Input: part model. Units: mm. Frame: model coordinates. A direction names the side the tool comes from. Coordinates: 2 decimals unless noted, no trailing zeros. Write each loop counter-clockwise with the first axis right and the second up, starting at its lowest first coordinate (ties: lowest second). Pieces come first, ordered by that corner, then holes. Notation, with made-up numbers: M -13.75,-23.75 L 7.25,-23.75 A25 ccw 7.25,0.25 Z; hole C 70,-13.5 d8. An arc over 180 degrees is marked long. Use one line per item in the form item = value.
from build123d import *

# Parameters (mm, degrees)
SKETCH1_W                                    = 70
SKETCH1_H                                    = 40
EXTRUDE1_DEPTH                               = 15
SKETCH3_R                                    = 20
EXTRUDE2_DEPTH                               = 10
SKETCH21_W                                   = 18
SKETCH21_H                                   = 45
EXTRUDE7_DEPTH                               = 15
F_25_0_MM_DOWEL_HOLES1_DEPTH                 = 15
F_25_0_MM_DOWEL_HOLES1_2_OUTLINE_R           = 12.5
F_25_0_MM_DOWEL_HOLES1_2_DEPTH               = 25
CSK_FOR_M5_COUNTERSUNK_FLAT_HEAD_SCR_2_COUNT = 2
CSK_FOR_M5_COUNTERSUNK_FLAT_HEAD_SCR_2_PITCH = 56
EXTRUDE8_START                               = -15
EXTRUDE8_DEPTH                               = 15
FILLET10_R                                   = 0.5
EXTRUDE9_DEPTH                               = 46.552167896
SKETCH23_W                                   = 2.5
SKETCH23_H                                   = 25
EXTRUDE10_DEPTH                              = 50.749371906
FILLET11_R                                   = 0.5
M6_CLEARANCE_HOLE1_D                         = 6.6


with BuildPart() as part:
    # Sketch1 → Extrude1 (new body)
    with BuildSketch(Plane(origin=(0, 0, 0), x_dir=(1, 0, 0), z_dir=(0, 1, 0))):
        Rectangle(SKETCH1_W, SKETCH1_H)
    extrude(amount=EXTRUDE1_DEPTH)

    # Sketch3 → Extrude2 (add)
    with BuildSketch(Plane(origin=(0, 15, 0), x_dir=(1, 0, 0), z_dir=(0, 1, 0))):
        with Locations(Location((0, 0, 0), (0, 0, 270))):
            Circle(SKETCH3_R)
    extrude(amount=EXTRUDE2_DEPTH)

    # 25.0 mm Dowel Holes1 2 outline → 25.0 mm Dowel Holes1 2 (cut)
    with BuildSketch(Plane(origin=(0, 0, 0), x_dir=(1, 0, 0), z_dir=(0, 1, 0))):
        Circle(F_25_0_MM_DOWEL_HOLES1_2_OUTLINE_R)
    extrude(amount=F_25_0_MM_DOWEL_HOLES1_2_DEPTH, mode=Mode.SUBTRACT)

    # Sketch11 → CSK for M5 Countersunk Flat Head Screw1 (revolve, cut)
    with BuildSketch(Plane(origin=(-28, 15, 0), x_dir=(0, 0, 1), z_dir=(1, 0, 0))):
        Polygon((0, 0), (0, 15), (5.2, 15), (2.75, 12.55), (2.75, 2.45), (5.2, 0), align=None)
    csk_for_m5_countersunk_flat_head_screw1 = revolve(axis=Axis((-28, 21.35, 0), (0, -1, 0)), mode=Mode.SUBTRACT)

    # CSK for M5 Countersunk Flat Head Scr 2: CSK for M5 Countersunk Flat Head Screw1 ×2
    with Locations(*[(i * CSK_FOR_M5_COUNTERSUNK_FLAT_HEAD_SCR_2_PITCH, 0, 0) for i in range(1, CSK_FOR_M5_COUNTERSUNK_FLAT_HEAD_SCR_2_COUNT)]):
        add(csk_for_m5_countersunk_flat_head_screw1, mode=Mode.SUBTRACT)


with BuildPart() as body_2:
    # Sketch21 → Extrude7 (new body)
    with BuildSketch(Plane.XZ):
        with Locations((0, 2.5)):
            Rectangle(SKETCH21_W, SKETCH21_H)
    extrude(amount=-EXTRUDE7_DEPTH)

    # Ø25.0 mm Dowel Holes1: read off the stored shape, not the designer's step
    # Ø25.0 mm Dowel Holes1 outline → Ø25.0 mm Dowel Holes1 (cut)
    with BuildSketch(Plane(origin=(0, 0, 0), x_dir=(1, 0, 0), z_dir=(0, 1, 0))):
        with BuildLine():
            Line((-9, 20), (-9, -8.674675786))
            ThreePointArc((-9, -8.674675786), (0, -12.5), (9, -8.674675786))
            Line((9, -8.674675786), (9, 20))
            Line((9, 20), (-9, 20))
        make_face()
    extrude(amount=F_25_0_MM_DOWEL_HOLES1_DEPTH, mode=Mode.SUBTRACT)


with BuildPart() as part_1:
    add(part.part)

    # Sculpt4: read off the stored shape, not the designer's step
    # Sculpt4: union body 2
    add(body_2.part)

    # Extrude8: read off the stored shape, not the designer's step
    # Extrude8 outline → Extrude8 (cut)
    with BuildSketch(Plane(origin=(0, 15, 0), x_dir=(1, 0, 0), z_dir=(0, 1, 0)).offset(EXTRUDE8_START)):
        Polygon((35, -20), (35, -7.150369323), (9, -17.919921944), (9, -20), align=None)
        with BuildLine():
            Line((-35, 20), (-35, 7.150369323))
            Line((-35, 7.150369323), (-7.653668647, 18.47759065))
            ThreePointArc((-7.653668647, 18.47759065), (-3.901806443, 19.615705608), (-6e-09, 20))
            Line((-6e-09, 20), (-35, 20))
        make_face()
        Polygon((-9, -20), (-9, -17.919921944), (-35, -7.150369323), (-35, -20), align=None)
        with BuildLine():
            Line((35, 20), (-6e-09, 20))
            ThreePointArc((-6e-09, 20), (3.901806437, 19.615705609), (7.653668647, 18.47759065))
            Line((7.653668647, 18.47759065), (35, 7.150369323))
            Line((35, 7.150369323), (35, 20))
        make_face()
    extrude(amount=EXTRUDE8_DEPTH, mode=Mode.SUBTRACT)

    # Fillet10
    fillet10_edges = [part_1.edges().sort_by_distance(p)[0] for p in [
        (0, 25, -20),
        (-12.5, 25, 0),
        (-35, 7.5, -7.150369323),
        (35, 7.5, -7.150369323),
        (35, 7.5, 7.150369323),
        (-35, 7.5, 7.150369323),
        (-9, 7.5, 25),
        (9, 7.5, 25),
    ]]
    fillet(fillet10_edges, radius=FILLET10_R)

    # Sketch22 → Extrude9 (cut, symmetric)
    with BuildSketch(Plane(origin=(0, 15, 0), x_dir=(1, 0, 0), z_dir=(0, 1, 0))):
        Polygon((-9, -149.154505921), (-9, -17.919921944), (-9, -15.919921944), (-13.828427125, -15.919921944), (-145.063011101, -15.919921944), (-328.697324176, -203.452594264), (-192.634313075, -336.68717824), align=None)
    extrude9 = extrude(amount=EXTRUDE9_DEPTH, both=True, mode=Mode.SUBTRACT)

    # Mirror3: Extrude9 across plane
    add(extrude9.mirror(Plane(origin=(0, 0, 0), x_dir=(0, 0, 1), z_dir=(1, 0, 0))), mode=Mode.SUBTRACT)

    # Sketch23 → Extrude10 (cut, through all)
    with BuildSketch(Plane.XZ):
        with Locations((0, 12.5)):
            Rectangle(SKETCH23_W, SKETCH23_H)
    extrude(amount=-EXTRUDE10_DEPTH, mode=Mode.SUBTRACT)

    # Fillet11
    fillet11_edges = [part_1.edges().sort_by_distance(p)[0] for p in [
        (-9, 12.5, 15.919921944),
        (-13.828427124, 7.5, 15.919921944),
        (13.828427124, 7.5, 15.919921944),
        (9, 12.5, 15.919921944),
    ]]
    fillet(fillet11_edges, radius=FILLET11_R)

    # M6 Clearance Hole1 (through all)
    with Locations(Plane.ZY.offset(9)):
        with Locations((20.704631923, 8.886572753)):
            Hole(M6_CLEARANCE_HOLE1_D / 2)


solid = part_1.part
(1) Pull-direction query (X, two-part tool) for faces 1 (the conical face through (-26.23, 12.7, -2.3)), 2 (the flat face through (24.5, 7.4, 11.5)), 3 (the flat face through (11, 13, 15.92)); classes: pulls with the +X half, pulls with the -X half, needs draft (parallel to the pull), parting line crosses it, or undercut.
Computed:
face_1 = undercut
face_2 = pulls with the +X half
face_3 = needs draft
(2) Set-up query: faces 4 (the flat face through (9, 10, 17)), 5 (the flat face through (5, 15, 22)), 6 (the flat face through (1.25, 12, 17)), 7 (the flat face through (20.983, 7.395, -12.956)). Return all of +Z, -Z, +X, -X, +Y, -Y with unobstructed straight access to the full face (end or side cutting, diameter ignored); none if empty.
Computed:
face_4 = +Z, +X, +Y, -Y
face_5 = +Z, +X, +Y
face_6 = +Z, +Y, -Y
face_7 = -Z, +X, +Y, -Y
(3) Section query A-A on x = -28. Return the cut outline in (y, z), plus the area to 3 significant figures.
Computed:
outline = M 0,-10.05 L 15,-10.05 L 15,-5.2 L 12.55,-2.75 L 2.45,-2.75 L 0,-5.2 Z; M 0,5.2 L 2.45,2.75 L 12.55,2.75 L 15,5.2 L 15,10.05 L 0,10.05 Z
area = 207 mm^2
(4) Section query B-B on y = 7.5. State how many separate pieces and enclosed holes the cut face has, plus the area to 3 significant figures.
Computed:
separate_pieces = 3
enclosed_holes = 2
area = 1,430 mm^2
(5) Line query: probe 1 along X at (y, z) = (5.5, 0); probe 2 along Y at (x, z) = (-1.5, 21); probe 3 along Z at (x, y) = (-30, 9.75). Output: solid intervals per line, ascending.
Computed:
probe_1 = -35 to -30.75, -25.25 to -12.5, 12.5 to 25.25, 30.75 to 35
probe_2 = 0 to 5.6, 12.17 to 15
probe_3 = -9.22 to -1.89, 1.89 to 9.22
(6) First-contact query: pin 1 Ø4 at (y, z) = (8.89, 20.7) entering from +X; pin 2 Ø1 at (x, y) = (27.5, 13) entering from +Z; pin 3 Ø5.5 at (x, z) = (-4, 22.5) entering from +Y; pin 4 Ø1.3 at (x, y) = (-12.5, 14.5) entering from +Z. Flat tips, straight axial feed; report the tip coordinate or a pass-through.
Computed:
pin_1 = through
pin_2 = 10.46
pin_3 = 15
pin_4 = 15.92
